Work out the finished part from the listing and answer in its coordinate system (mm). Coordinates: 2 decimals unless noted, no trailing zeros. Loops run counter-clockwise (first coordinate to the right, second up) from the corner with the lowest first, then second, coordinate; pieces in that order, holes last. Notation, with made-up numbers: (33, -13) -> (88, -13) arc R23 ccw to (88, 23) -> close; hole circle Ø5 at (74, -1). An arc over 180 degrees is marked (long way). One line per question, with ' | ' between items.
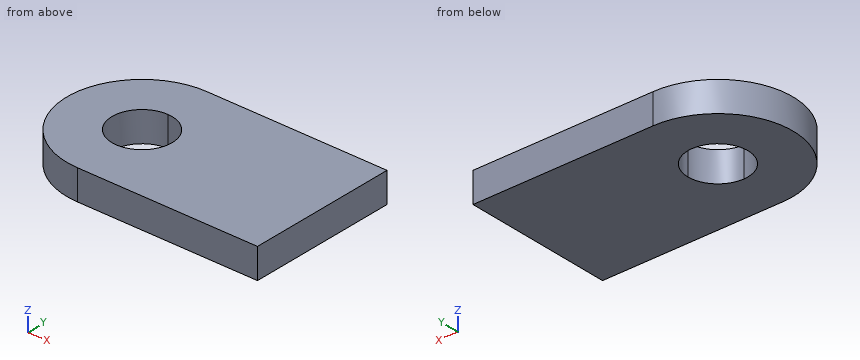
```python
from build123d import *

# Parameters (mm, degrees)
F1_DEPTH = 12.7


# Not quite as in the source:
# - a feature of the source that left no trace in its solid (it failed there, or was rolled back) is left out


with BuildPart() as f1:
    # F0 (on Top) → F1 (new body)
    with BuildSketch(Plane.XY):
        with BuildLine():
            Line((-38.1, -31.75), (38.1, -31.75))
            Line((38.1, -31.75), (38.1, 31.75))
            Line((38.1, 31.75), (-38.1, 31.75))
            ThreePointArc((-38.1, 31.75), (-15.6493596973, 22.4506403027), (-6.35, 0))
            ThreePointArc((-6.35, 0), (-15.6493596973, -22.4506403027), (-38.1, -31.75))
        make_face()
        with BuildLine():
            ThreePointArc((-38.1, 31.75), (-69.85, 0), (-38.1, -31.75))
            Line((-38.1, -31.75), (-38.1, -12.7))
            ThreePointArc((-38.1, -12.7), (-50.8, 0), (-38.1, 12.7))
            Line((-38.1, 12.7), (-38.1, 31.75))
        make_face()
        with BuildLine():
            Line((-38.1, -12.7), (-38.1, -31.75))
            ThreePointArc((-38.1, -31.75), (-15.6493596973, -22.4506403027), (-6.35, 0))
            ThreePointArc((-6.35, 0), (-15.6493596973, 22.4506403027), (-38.1, 31.75))
            Line((-38.1, 31.75), (-38.1, 12.7))
            ThreePointArc((-38.1, 12.7), (-29.1197438789, 8.9802561211), (-25.4, 0))
            ThreePointArc((-25.4, 0), (-29.1197438789, -8.9802561211), (-38.1, -12.7))
        make_face()
    extrude(amount=F1_DEPTH)


solid = f1.part
```
1) Find the intervals of material crossed by line 1 along X through (y, z) = (-8.5, 8.75); line 2 along X through (y, z) = (10, 10.75); line 3 along X through (y, z) = (25.5, 5.5), in increasing order.
Check values:
line 1: x = -68.69 to -47.54, -28.66 to 38.1 | line 2: x = -68.23 to -45.93, -30.27 to 38.1 | line 3: x = -57.02 to 38.1
2) Find section B-B (y = -7). Write down the section's boundary in (x, z).
Check values:
outline: (-69.07, 0) -> (-48.7, 0) -> (-48.7, 12.7) -> (-69.07, 12.7) -> close; (-27.5, 0) -> (38.1, 0) -> (38.1, 12.7) -> (-27.5, 12.7) -> close
3) Find section A-A (z = 6.75). Write down the section's boundary in (x, y), plus the area to 3 significant figures.
Check values:
outline: (-38.1, -31.75) -> (38.1, -31.75) -> (38.1, 31.75) -> (-38.1, 31.75) arc R31.75 ccw to start; hole circle Ø25.4 at (-38.1, 0) | area: 5,920 mm^2
4) Find section C-C (x = -35.5). Write down the section's boundary in (y, z), plus the area to 3 significant figures.
Check values:
outline: (-31.75, 0) -> (-12.43, 0) -> (-12.43, 12.7) -> (-31.75, 12.7) -> close; (12.43, 0) -> (31.75, 0) -> (31.75, 12.7) -> (12.43, 12.7) -> close | area: 491 mm^2
5) Find section D-D (y = 24). Write down the section's boundary in (x, z).
Check values:
outline: (-58.89, 0) -> (38.1, 0) -> (38.1, 12.7) -> (-58.89, 12.7) -> close
6) A flat-ended cylindrical pin translates along its axis: pin 1 (5 mm diameter, centred on y = -21, z = 7, fed in from -X). Find the tip coordinate at first contact, or state that the pin passes through.
Check values:
pin 1: stops at x = -63.9
